```python
from build123d import *

# Parameters (mm, degrees)
F0_W     = 86.47044
F0_H     = 64.107388
F1_DEPTH = 25.4
F2_R     = 16.446559
F3_DEPTH = 25.4
F5_DEPTH = 64.108388


with BuildPart() as f1:
    # F0 (on Right) → F1 (new body)
    with BuildSketch(Plane.YZ):
        Rectangle(F0_W, F0_H)
    extrude(amount=F1_DEPTH)

    # F2 (on face) → F3 (join)
    with BuildSketch(Plane.YZ.offset(25.4)):
        Circle(F2_R)
    extrude(amount=F3_DEPTH)

    # F4 (on face) → F5 (cut, through all)
    with BuildSketch(Plane(origin=(0, 0, -32.053694), x_dir=(1, 0, 0), z_dir=(0, 0, -1))):
        Polygon((50.8, -16.446559), (50.8, 16.446559), (25.4, -16.446559), align=None)
    extrude(amount=-F5_DEPTH, mode=Mode.SUBTRACT)


solid = f1.part
```
Part model, mm, in its own coordinate system. Coordinates: 2 decimals unless noted, no trailing zeros. Write each loop counter-clockwise with the first axis right and the second up, starting at its lowest first coordinate (ties: lowest second). Pieces come first, ordered by that corner, then holes.
Item 1: Slice it at B-B (z = 2). Write the cut outline in (x, y).
Item 2: Probe line 1 (X direction, y = -38, z = 9.5); line 2 (X direction, y = 15.5, z = -1.5); line 3 (Y direction, x = 41, z = -14.5). List the from-to ranges inside material, lowest first.
Item 3: Slice it at C-C (x = 43). Write the cut outline in (y, z).
Item 4: Pin check, flat tips, straight feed: pin 1 (5 mm diameter, centred on x = 39.5, z = -8.5, fed in from -Y); pin 2 (1 mm diameter, centred on y = -20.5, z = -14, fed in from +X); pin 3 (3 mm diameter, centred on y = -7.5, z = 2, fed in from +X). Stop position of each tip, or through.
Item 5: Slice it at A-A (y = 0). Write the cut outline in (x, z).
Item 6: Slice it at D-D (y = 37). Write the cut outline in (x, z), and give its area (3 significant figures).
Results found:
1. outline: (0, -43.24) - (25.4, -43.24) - (25.4, -16.32) - (50.71, -16.32) - (25.49, 16.32) - (25.4, 16.32) - (25.4, 43.24) - (0, 43.24) - close
2. line 1: x = 0 to 25.4
2. line 2: x = 0 to 26.13
2. line 3: y = -7.76 to -3.76
3. outline: (-6.35, -15.17) - (-6.35, 15.17) arc R16.45 ccw to start
4. pin 1: stops at y = -15.31
4. pin 2: stops at x = 25.4
4. pin 3: stops at x = 45.05
5. outline: (0, -32.05) - (25.4, -32.05) - (25.4, -16.45) - (38.1, -16.45) - (38.1, 16.45) - (25.4, 16.45) - (25.4, 32.05) - (0, 32.05) - close
6. outline: (0, -32.05) - (25.4, -32.05) - (25.4, 32.05) - (0, 32.05) - close
6. area: 1,630 mm2
